from build123d import *

# Parameters (mm, degrees)
ESQUISSE1_W             = 30
ESQUISSE1_H             = 25
BOSS_EXTRU_1_DEPTH      = 5
ESQUISSE2_W             = 28
ESQUISSE2_H             = 23
ENL_V_MAT_EXTRU_1_DEPTH = 4
ESQUISSE3_W             = 3.35
ESQUISSE3_H             = 10
ENL_V_MAT_EXTRU_2_DEPTH = 10
ESQUISSE4_W             = 4
ESQUISSE4_H             = 23
ENL_V_MAT_EXTRU_3_DEPTH = 10
BOSS_EXTRU_2_DEPTH      = 3.5
CONG_3_R                = 0.5
ENL_V_MAT_EXTRU_6_DEPTH = 0.5
ESQUISSE12_W            = 7
ESQUISSE12_H            = 25
BOSS_EXTRU_5_DEPTH      = 0.5
CONG_5_R                = 0.5
ESQUISSE13_R            = 0.5
ENL_V_MAT_EXTRU_8_DEPTH = 10.5


with BuildPart() as part:
    # Esquisse1 → Boss.-Extru.1 (new body)
    with BuildSketch(Plane.XY):
        with Locations((15, 12.5)):
            Rectangle(ESQUISSE1_W, ESQUISSE1_H)
    extrude(amount=BOSS_EXTRU_1_DEPTH)

    # Esquisse2 → Enlèv. mat.-Extru.1 (cut)
    with BuildSketch(Plane.XY.offset(5)):
        with Locations((15, 12.5)):
            Rectangle(ESQUISSE2_W, ESQUISSE2_H)
    extrude(amount=-ENL_V_MAT_EXTRU_1_DEPTH, mode=Mode.SUBTRACT)

    # Esquisse3 → Enlèv. mat.-Extru.2 (cut)
    with BuildSketch(Plane.ZY):
        with Locations((3.325, 12.5)):
            Rectangle(ESQUISSE3_W, ESQUISSE3_H)
    extrude(amount=-ENL_V_MAT_EXTRU_2_DEPTH, mode=Mode.SUBTRACT)

    # Esquisse4 → Enlèv. mat.-Extru.3 (cut)
    with BuildSketch(Plane(origin=(30, 0, 0), x_dir=(0, 0, -1), z_dir=(1, 0, 0))):
        with Locations((-3, 12.5)):
            Rectangle(ESQUISSE4_W, ESQUISSE4_H)
    extrude(amount=-ENL_V_MAT_EXTRU_3_DEPTH, mode=Mode.SUBTRACT)

    # Esquisse5 → Boss.-Extru.2 (add)
    # profile 1 of 2: a face of its own
    with BuildSketch(Plane.XY.offset(1)):
        with BuildLine():
            Line((19.311805698, 24.2), (22.688194302, 24.2))
            ThreePointArc((22.688194302, 24.2), (21, 22.3), (19.311805698, 24.2))
        make_face()
        with BuildLine():
            Line((19.5, 24), (22.5, 24))
            ThreePointArc((22.5, 24), (21, 22.5), (19.5, 24))
        make_face(mode=Mode.SUBTRACT)
    # profile 2 of 2: a face of its own
    with BuildSketch(Plane.XY.offset(1)):
        with BuildLine():
            Line((19.311805698, 0.8), (22.688194302, 0.8))
            ThreePointArc((22.688194302, 0.8), (21, 2.7), (19.311805698, 0.8))
        make_face()
        with BuildLine():
            Line((19.5, 1), (22.5, 1))
            ThreePointArc((22.5, 1), (21, 2.5), (19.5, 1))
        make_face(mode=Mode.SUBTRACT)
    extrude(amount=BOSS_EXTRU_2_DEPTH)

    # Congé3
    cong_3_edges = [part.edges().sort_by_distance(p)[0] for p in [
        (15, 25, 0),
        (15, 0, 0),
        (0, 12.5, 0),
        (0, 25, 2.5),
        (0, 0, 2.5),
    ]]
    fillet(cong_3_edges, radius=CONG_3_R)

    # Esquisse9 → Enlèv. mat.-Extru.6 (cut)
    with BuildSketch(Plane.XY.offset(5)):
        Polygon((0.2, 7.5), (0.2, 0.2), (30, 0.2), (30, 1), (1, 1), (1, 7.5), align=None)
        Polygon((1, 17.5), (0.2, 17.5), (0.2, 24.8), (30, 24.8), (30, 24), (1, 24), align=None)
    extrude(amount=-ENL_V_MAT_EXTRU_6_DEPTH, mode=Mode.SUBTRACT)

    # Esquisse12 → Boss.-Extru.5 (add)
    with BuildSketch(Plane(origin=(30, 0, 0), x_dir=(0, 0, -1), z_dir=(1, 0, 0))):
        with Locations((-3.5, 12.5)):
            Rectangle(ESQUISSE12_W, ESQUISSE12_H)
    extrude(amount=BOSS_EXTRU_5_DEPTH)

    # Congé5
    # the kernel refuses this fillet: 0.5 mm, written as the material it takes off along each edge
    with BuildSketch(Plane(origin=(30, 0.5, 0.5), x_dir=(0, 0, -1), z_dir=(0, -1, 0))) as cong_5_piece_1_section:
        Polygon((0, 0), (CONG_5_R * 1.02, 0), (CONG_5_R * 1.02, CONG_5_R * 1.02), (0, CONG_5_R * 1.02), align=None)
    cong_5_piece_1 = extrude(amount=CONG_5_R * 1.02, mode=Mode.PRIVATE)
    cong_5_piece_1 = cong_5_piece_1 - Plane(origin=(30, 0.5, 0.5), x_dir=(-0.7071067811865475, 0, 0.7071067811865475), z_dir=(0, -1, 0)) * Sphere(CONG_5_R, mode=Mode.PRIVATE)
    add(cong_5_piece_1, mode=Mode.SUBTRACT)
    with BuildSketch(Plane(origin=(30, 24.5, 0.5), x_dir=(1, 0, 0), z_dir=(0, 0, -1))) as cong_5_piece_2_section:
        Polygon((0, 0), (CONG_5_R * 1.02, 0), (CONG_5_R * 1.02, -CONG_5_R * 1.02), (0, -CONG_5_R * 1.02), align=None)
    cong_5_piece_2 = extrude(amount=CONG_5_R * 1.02, mode=Mode.PRIVATE)
    cong_5_piece_2 = cong_5_piece_2 - Plane(origin=(30, 24.5, 0.5), x_dir=(-0.7071067811865475, -0.7071067811865475, 0), z_dir=(0, 0, -1)) * Sphere(CONG_5_R, mode=Mode.PRIVATE)
    add(cong_5_piece_2, mode=Mode.SUBTRACT)
    with BuildSketch(Plane(origin=(30.5, 24.5, 0), x_dir=(-1, 0, 0), z_dir=(0, -1, 0))) as cong_5_piece_3:
        with BuildLine():
            CenterArc((CONG_5_R, -CONG_5_R), CONG_5_R, 90, 90)
            Line((0, -CONG_5_R), (0, 0))
            Line((0, 0), (CONG_5_R, 0))
        make_face()
    extrude(amount=24, mode=Mode.SUBTRACT)
    with BuildSketch(Plane(origin=(30.5, 25, 8.25), x_dir=(0, -1, 0), z_dir=(0, 0, -1))) as cong_5_piece_4:
        with BuildLine():
            CenterArc((CONG_5_R, CONG_5_R), CONG_5_R, 180, 90)
            Line((0, CONG_5_R), (0, 0))
            Line((0, 0), (CONG_5_R, 0))
        make_face()
    extrude(amount=7.75, mode=Mode.SUBTRACT)
    with BuildSketch(Plane(origin=(30.5, 0, 0.5), x_dir=(-1, 0, 0), z_dir=(0, 0, 1))) as cong_5_piece_5:
        with BuildLine():
            CenterArc((CONG_5_R, -CONG_5_R), CONG_5_R, 90, 90)
            Line((0, -CONG_5_R), (0, 0))
            Line((0, 0), (CONG_5_R, 0))
        make_face()
    extrude(amount=7.75, mode=Mode.SUBTRACT)

    # Esquisse13 → Enlèv. mat.-Extru.8 (cut)
    with BuildSketch(Plane(origin=(0, 0, 0), x_dir=(-1, 0, 0), z_dir=(0, 0, -1))):
        with Locations((-26, 19.5)):
            Circle(ESQUISSE13_R)
        with Locations((-16, 19.5)):
            Circle(ESQUISSE13_R)
        with Locations((-6, 19.5)):
            Circle(ESQUISSE13_R)
        with Locations((-16, 14.5)):
            Circle(ESQUISSE13_R)
        with Locations((-6, 14.5)):
            Circle(ESQUISSE13_R)
        with Locations((-16, 9.5)):
            Circle(ESQUISSE13_R)
        with Locations((-6, 9.5)):
            Circle(ESQUISSE13_R)
        with Locations((-16, 4.5)):
            Circle(ESQUISSE13_R)
        with Locations((-6, 4.5)):
            Circle(ESQUISSE13_R)
        with Locations((-26, 14.5)):
            Circle(ESQUISSE13_R)
        with Locations((-26, 9.5)):
            Circle(ESQUISSE13_R)
        with Locations((-26, 4.5)):
            Circle(ESQUISSE13_R)
    extrude(amount=-ENL_V_MAT_EXTRU_8_DEPTH, mode=Mode.SUBTRACT)


solid = part.part
Read the model definition and answer for the solid it produces. Units are mm, in the model's axes. A direction names the side the tool comes from. Round coordinates to 2 decimals unless told otherwise and drop trailing zeros. Write each loop counter-clockwise with the first axis right and the second up, starting at its lowest first coordinate (ties: lowest second). Pieces come first, ordered by that corner, then holes. Notation, with made-up numbers: M 83.25,-7.75 L 119.25,-7.75 A36 cw 119.25,27.25 Z; hole C -31,41 d7. An arc over 180 degrees is marked long. Use a Markdown table: item, result.
1) The part is cut by section B-B (x = 26). Give the number of separate pieces and of enclosed holes in the cut face, plus the area to 3 significant figures.
Answers follow:
| item | result |
|---|---|
| separate pieces | 5 |
| enclosed holes | 0 |
| area | 28.1 mm2 |
2) The part is cut by section A-A (y = 14.5). Write down the section's boundary in (x, z).
Answers follow:
| item | result |
|---|---|
| outline | M 0,0.5 A0.5 ccw 0.5,0 L 5.5,0 L 5.5,1 L 1,1 L 1,1.65 L 0,1.65 Z; M 6.5,0 L 15.5,0 L 15.5,1 L 6.5,1 Z; M 16.5,0 L 25.5,0 L 25.5,1 L 16.5,1 Z; M 26.5,0 L 30,0 A0.5 ccw 30.5,0.5 L 30.5,7 L 30,7 L 30,1 L 26.5,1 Z |
3) The part is cut by section D-D (x = 21). Write down the section's boundary in (y, z).
Answers follow:
| item | result |
|---|---|
| outline | M 0,0.5 A0.5 ccw 0.5,0 L 24.5,0 A0.5 ccw 25,0.5 L 25,5 L 24.8,5 L 24.8,4.5 L 24,4.5 L 24,1 L 22.5,1 L 22.5,4.5 L 22.3,4.5 L 22.3,1 L 2.7,1 L 2.7,4.5 L 2.5,4.5 L 2.5,1 L 1,1 L 1,4.5 L 0.2,4.5 L 0.2,5 L 0,5 Z |
4) A tool of negligible diameter and unlimited length cuts with its end or side. For faces 4 (the flat face through (26, 1, 3)), 5 (the cylindrical face through (16.065, 19.996, 0.493)), 6 (the flat face through (0.5, 12.4, 1.65)), from which of +Z, -Z, +X, -X, +Y, -Y can it reach the whole face along a straight path? Write none if from no direction.
Answers follow:
| item | result |
|---|---|
| face 4 | +Z |
| face 5 | +Z, -Z |
| face 6 | +Z, -X |
5) For a pull along Y with two mould halves and no side action, classify faces 1 (the flat face through (15, 0, 3)), 2 (the flat face through (11.9, 24.4, 4.5)), 3 (the flat face through (0, 12, 1)) as pulls with the +Y half, pulls with the -Y half, needs draft (parallel to the pull), parting line crosses it, or undercut.
Answers follow:
| item | result |
|---|---|
| face 1 | pulls with the -Y half |
| face 2 | undercut |
| face 3 | needs draft |
6) A flat-ended cylindrical pin translates along its axis: pin 1 (6 mm diameter, centred on x = 17.5, y = 2.5, fed in from +Z). Find the tip coordinate at first contact, or state that the pin passes through.
Answers follow:
| item | result |
|---|---|
| pin 1 | stops at z = 5 |
7) The part is cut by section C-C (z = 4). Write down the section's boundary in (x, y), plus the area to 3 significant figures.
Answers follow:
| item | result |
|---|---|
| outline | M 0,0.5 A0.5 ccw 0.5,0 L 30,0 A0.5 ccw 30.5,0.5 L 30.5,24.5 A0.5 ccw 30,25 L 0.5,25 A0.5 ccw 0,24.5 L 0,17.5 L 1,17.5 L 1,24 L 19.3,24 A1.7 ccw 22.7,24 L 30,24 L 30,1 L 22.7,1 A1.7 ccw 19.3,1 L 1,1 L 1,7.5 L 0,7.5 Z; hole M 19.5,1 L 22.5,1 A1.5 ccw Z; hole M 19.5,24 A1.5 ccw 22.5,24 Z |
| area | 87.3 mm2 |
8) Straight lines are drawn through the part: line 1 along Y through (x, z) = (26, 0.55); line 2 along X through (y, z) = (19, 4); line 3 along Y through (x, z) = (21.5, 3). For each, find the intervals that lie inside material, in ascending order. Write a range as [from, to].
Answers follow:
| item | result |
|---|---|
| line 1 | y = [0, 4], [5, 9], [10, 14], [15, 19], [20, 25] |
| line 2 | x = [0, 1], [30, 30.5] |
| line 3 | y = [0, 1], [2.41, 2.62], [22.38, 22.59], [24, 25] |
